Can you work these out from the model? Positions are in its coordinate system, mm. Face numbers are marked on the shaded views. A direction names the side the tool comes from. Round coordinates to 2 decimals unless told otherwise and drop trailing zeros. Write each loop counter-clockwise with the first axis right and the second up, starting at its lowest first coordinate (ties: lowest second). Pieces come first, ordered by that corner, then holes. Notation, with made-up numbers: (28.5, 37.25) -> (57.5, 37.25) arc R12 cw to (57.5, 54.25) -> close; hole circle Ø1 at (79.25, 39.25). An arc over 180 degrees is marked (long way). Use CSV: the item, a comma, the result in double quotes.
```python
from build123d import *

# Parameters (mm, degrees)
F0_R           = 25.4
F1_DEPTH       = 76.2
F3_D           = 17.5
F3_CBORE_D     = 25.5
F3_CBORE_DEPTH = 16
F4_R           = 5.08


with BuildPart() as f1:
    # F0 (on Top) → F1 (new body)
    with BuildSketch(Plane.XY):
        Circle(F0_R)
    extrude(amount=F1_DEPTH)

    # F3 (through all)
    with Locations(Plane.XY.offset(76.2)):
        with Locations((0, 0)):
            CounterBoreHole(F3_D / 2, F3_CBORE_D / 2, F3_CBORE_DEPTH)

    # F4
    f4_edges = [f1.edges().sort_by_distance(p)[0] for p in [
        (-25.4, 0, 76.2),
        (-25.4, 0, 0),
    ]]
    fillet(f4_edges, radius=F4_R)


solid = f1.part
```
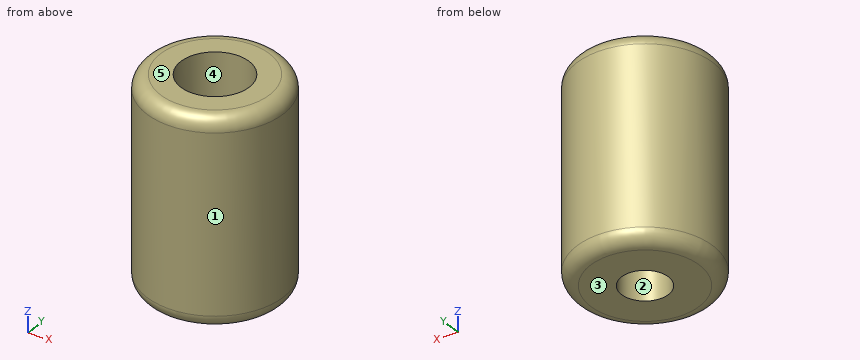
Q1. Suppose I cut it at A-A (x = 0). Write out the boundary of the cut face in (y, z), and give its area (3 significant figures).
Resolved:
outline,"(-25.4, 5.08) arc R5.08 ccw to (-20.32, 0) -> (-8.75, 0) -> (-8.75, 60.2) -> (-12.75, 60.2) -> (-12.75, 76.2) -> (-20.32, 76.2) arc R5.08 ccw to (-25.4, 71.12) -> close; (8.75, 0) -> (20.32, 0) arc R5.08 ccw to (25.4, 5.08) -> (25.4, 71.12) arc R5.08 ccw to (20.32, 76.2) -> (12.75, 76.2) -> (12.75, 60.2) -> (8.75, 60.2) -> close"
area,"2,390 mm^2"
Q2. Will these pins go through, and if not, where does the flat tip stop? P1, Ø6, axis at x = -20, z = 48, coming from the +Y side; P2, Ø2, axis at y = 9, z = 30, coming from the +X side; P3, Ø1.5, axis at x = -13.5, z = 22.5, coming from the -Y side.
Resolved:
P1,"stops at y = 18.87"
P2,"stops at x = 24.11"
P3,"stops at y = -21.97"
Q3. Please list where these lines run through material, in increasing order: probe 1 along Y at (x, z) = (0, 63.75); probe 2 along Y at (x, z) = (0, 18.5); probe 3 along X at (y, z) = (0.5, 39).
Resolved:
probe 1,"y = -25.4 to -12.75, 12.75 to 25.4"
probe 2,"y = -25.4 to -8.75, 8.75 to 25.4"
probe 3,"x = -25.4 to -8.74, 8.74 to 25.4"
Q4. Suppose I cut it at C-C (z = 38). Write out the boundary of the cut face in (x, y).
Resolved:
outline,"circle Ø50.8 at (0, 0); hole circle Ø17.5 at (0, 0)"
Q5. On a 3-axis mill with a long thin cutter (end or side, diameter ignored), from which of +Z, -Z, +X, -X, +Y, -Y can I reach the whole of each face in a straight line? I mean the marked faces 4 and 5. Say none if no direction works.
Resolved:
face 4,"+Z"
face 5,"+Z, +X, -X, +Y, -Y"
Q6. If we mould it in two halves opening along X, with no side actions, what happens to the marked faces 1, 2 and 3? For each: released by +X, released by -X, zero draft, split by the parting line, or undercut.
Resolved:
face 1,"split by the parting line"
face 2,"undercut"
face 3,"zero draft"
